```python
from build123d import *

# Parameters (mm, degrees)
F2_R     = 1.5875
F3_DEPTH = 9.525
F4_R     = 1.5875


with BuildPart() as f1:
    # F0 (on Front) → F1 (revolve)
    with BuildSketch(Plane.XZ):
        Polygon((5.0038, 0), (0, 0), (0, -11.1252), (2.38125, -11.1252), (2.69875, -11.1252), (2.69875, -7.9502), (2.38125, -7.9502), (2.38125, -1.6002), (5.0038, -1.6002), align=None)
    revolve(axis=Axis((0, 0, -5.5626), (0, 0, 1)))

    # F2 (on face) → F3 (cut)
    with BuildSketch(Plane.XY):
        Circle(F2_R)
    extrude(amount=-F3_DEPTH, mode=Mode.SUBTRACT)

    # F4
    f4_edges = [f1.edges().sort_by_distance(p)[0] for p in [
        (-5.0038, 0, 0),
    ]]
    fillet(f4_edges, radius=F4_R)


with BuildPart() as f1_1:
    # F5: moved
    add(f1.part.moved(Location((0, 0, 1.5875))))


solid = f1_1.part
```
The model under review builds one solid part; all positions refer to its coordinate system, in mm. A direction names the side the tool comes from. Coordinates: 2 decimals unless noted, no trailing zeros. Order: outer loops, then holes, each group sorted by start corner. A loop starts at its lowest first (then second) coordinate and runs counter-clockwise, first axis right, second up. Notation, with made-up numbers: (35, 46.5) -> (46, 46.5) arc R15 cw to (46, 62.5) -> close; hole circle Ø11 at (11.5, -9). An arc over 180 degrees is marked (long way). Answer in a Markdown table with one row per item. Add a question column.
Item 1: Clearance check with flat-ended pins moving along their axes: pin 1 (1.5 mm diameter, centred on y = -0.5, z = -7.5, fed in from +X); pin 2 (5 mm diameter, centred on y = -1.5, z = -3.5, fed in from -X); pin 3 (1.6 mm diameter, centred on x = 0, y = 0, fed in from +Z). State where each tip first meets the part, or that it passes through.
Item 2: Mouldability with a two-part tool opening along X and no side actions: class faces 4 (the cylindrical face through (-1.99, 1.82, -7.93)), 5 (the flat face through (0, 0, -7.938)), 6 (the flat face through (0, 0, -9.538)) as +X half, -X half, draft (parallel to the pull), parting line (faces both ways), or undercut.
Item 3: To check wall thickness, follow probe 1 along Y at (x, z) = (0, -4.75); probe 2 along Z at (x, y) = (-1.25, 3); probe 3 along Y at (x, z) = (0.75, -6). State the ranges of each line that lie inside material, in increasing order.
Item 4: We need section D-D on z = -2.5. Write out the cut boundary in (x, y) (1 decimal), plus the area to 3 significant figures.
Item 5: We need section C-C on z = 0.5. Write out the cut boundary in (x, y) (1 decimal).
Item 6: Machinability: for faces 1 (the flat face through (-2, -1, 1.588)), 2 (the cylindrical face through (-0.34, -1.55, -3.11)), 3 (the cylindrical face through (-1.89, -1.45, -3.14)), which of the approach directions +Z, -Z, +X, -X, +Y, -Y give a long, thin tool a straight path to every point of the face, cutting with its end or side? Answer none if there is none.
Final values:
| question | item | result |
|---|---|---|
| 1 | pin 1 | stops at x = 2.7 |
| 1 | pin 2 | stops at x = -2.38 |
| 1 | pin 3 | stops at z = -7.94 |
| 2 | face 4 | parting line |
| 2 | face 5 | undercut |
| 2 | face 6 | draft |
| 3 | probe 1 | y = -2.38 to -1.59, 1.59 to 2.38 |
| 3 | probe 2 | z = -0.01 to 1.59 |
| 3 | probe 3 | y = -2.26 to -1.4, 1.4 to 2.26 |
| 4 | outline | circle Ø4.8 at (0, 0); hole circle Ø3.2 at (0, 0) |
| 4 | area | 9.90 mm2 |
| 5 | outline | circle Ø9.8 at (0, 0); hole circle Ø3.2 at (0, 0) |
| 6 | face 1 | +Z, +X, -X, +Y, -Y |
| 6 | face 2 | +Z |
| 6 | face 3 | none |
